```python
from build123d import *

# Parameters (mm, degrees)
EKSTR_ZYON_NCE1_DEPTH       = 12.5
IZIM2_R                     = 1
KES_EKSTR_ZYON1_DEPTH       = 2
IZIM3_W                     = 3.969414418
IZIM3_H                     = 2.023180186
KES_EKSTR_ZYON2_DEPTH       = 3
IZIM4_R                     = 9.625
IZIM4_R_2                   = 8.125
Y_KSEKLIK_EKSTR_ZYON1_DEPTH = 5


with BuildPart() as part:
    # Çizim1 → Ekstrüzyon-İnce1 (new body)
    with BuildSketch(Plane.XY):
        Polygon((28.3, 0), (23.3, 0), (23.3, 16.15), (0, 16.15), (0, 0), (-5, 0), (-5, 1), (-1, 1), (-1, 17.15), (24.3, 17.15), (24.3, 1), (28.3, 1), align=None)
    extrude(amount=EKSTR_ZYON_NCE1_DEPTH)

    # Çizim2 → Kes-Ekstrüzyon1 (cut, through all)
    with BuildSketch(Plane(origin=(0, 1, 0), x_dir=(1, 0, 0), z_dir=(0, 1, 0))):
        with Locations((-2.85, -6.25)):
            Circle(IZIM2_R)
        with Locations((26.15, -6.25)):
            Circle(IZIM2_R)
    extrude(amount=-KES_EKSTR_ZYON1_DEPTH, mode=Mode.SUBTRACT)

    # Çizim3 → Kes-Ekstrüzyon2 (cut)
    with BuildSketch(Plane.ZY.offset(1)):
        with Locations((6.240510002, 10.825173076)):
            Rectangle(IZIM3_W, IZIM3_H)
    extrude(amount=-KES_EKSTR_ZYON2_DEPTH, mode=Mode.SUBTRACT)

    # Çizim4 → Yükseklik-Ekstrüzyon1 (add)
    with BuildSketch(Plane(origin=(0, 17.15, 0), x_dir=(1, 0, 0), z_dir=(0, 1, 0))):
        with Locations((11.64, -6.25)):
            Circle(IZIM4_R)
        with Locations((11.64, -6.25)):
            Circle(IZIM4_R_2, mode=Mode.SUBTRACT)
    extrude(amount=Y_KSEKLIK_EKSTR_ZYON1_DEPTH)


solid = part.part
```
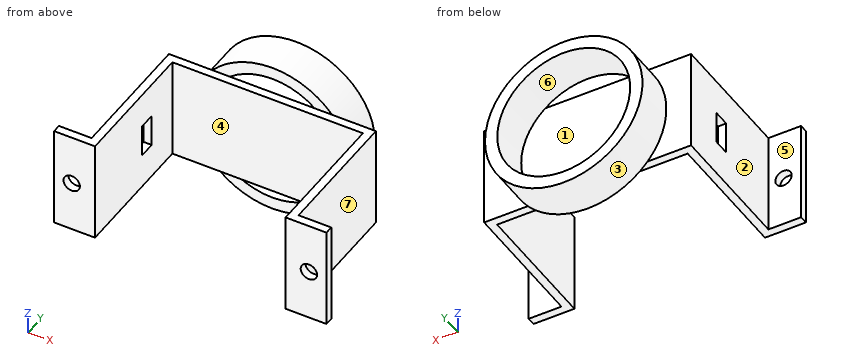
Source: CAD feature listing. Evaluate the final solid. Frame: model axes, mm. Face numbers are marked on the shaded views. A direction names the side the tool comes from. Round coordinates to 2 decimals unless told otherwise and drop trailing zeros. Loops run counter-clockwise (first coordinate to the right, second up) from the corner with the lowest first, then second, coordinate; pieces in that order, holes last.
1. Ray query, L1, parallel to X at y = 0.6, z = 6.25; L2, parallel to Z at x = 26.15, y = 0.6; L3, parallel to X at y = 13.25, z = 11.5. Return the intervals inside material, ascending.
2. Contact query for flat-ended pins moving along their axis: pin 1 (4 mm diameter, centred on x = 13, z = 6.5, fed in from +Y); pin 2 (1.5 mm diameter, centred on x = 17, z = 1, fed in from -Y); pin 3 (6 mm diameter, centred on y = 9.5, z = 3.5, fed in from -X). Output: stop coordinate, or through.
3. Section query D-D on y = 6. Output: boundary loops of the cut face in (x, z).
4. Mould query, pull axis Z, two halves, no side actions, for the marked faces 1, 2 and 3. Classes: released by +Z, released by -Z, zero draft, split by the parting line, or undercut.
5. Section query C-C on x = -2.85. Output: boundary loops of the cut face in (y, z), and give its area (3 significant figures).
6. Access query for the marked faces 4, 5, 6 and 7. Directions: +Z, -Z, +X, -X, +Y, -Y. A direction counts if a zero-diameter tool reaches every point of the face in a straight line with its end or side. Return the directions, or none.
7. Section query B-B on y = 10.5. Output: boundary loops of the cut face in (x, z).
8. Section query A-A on x = 11.64. Output: boundary loops of the cut face in (y, z) (3 decimals).
Answers below:
1. L1: x = -5 to -3.85, -1.85 to 0, 23.3 to 25.15, 27.15 to 28.3
1. L2: z = 0 to 5.25, 7.25 to 12.5
1. L3: x = -1 to 0, 23.3 to 24.3
2. pin 1: stops at y = 17.15
2. pin 2: stops at y = 16.15
2. pin 3: stops at x = -1
3. outline: (-1, 0) - (0, 0) - (0, 12.5) - (-1, 12.5) - close; (23.3, 0) - (24.3, 0) - (24.3, 12.5) - (23.3, 12.5) - close
4. face 1: undercut
4. face 2: zero draft
4. face 3: split by the parting line
5. outline: (0, 0) - (1, 0) - (1, 5.25) - (0, 5.25) - close; (0, 7.25) - (1, 7.25) - (1, 12.5) - (0, 12.5) - close
5. area: 10.5 mm2
6. face 4: +Z, -Z, -Y
6. face 5: +Z, -Z, -X, +Y
6. face 6: +Y
6. face 7: +Z, -Z, +X, +Y
7. outline: (-1, 0) - (0, 0) - (0, 4.26) - (-1, 4.26) - close; (-1, 8.23) - (0, 8.23) - (0, 12.5) - (-1, 12.5) - close; (23.3, 0) - (24.3, 0) - (24.3, 12.5) - (23.3, 12.5) - close
8. outline: (16.15, 0) - (17.15, 0) - (17.15, 12.5) - (16.15, 12.5) - close; (17.15, -3.375) - (22.15, -3.375) - (22.15, -1.875) - (17.15, -1.875) - close; (17.15, 14.375) - (22.15, 14.375) - (22.15, 15.875) - (17.15, 15.875) - close
